The listing builds one solid part. Answer for the finished solid, in the listing's coordinates (mm). Face numbers are marked on the shaded views. Give positions to 0.01 mm unless a question says otherwise; leave off trailing zeros. Order: outer loops, then holes, each group sorted by start corner. A loop starts at its lowest first (then second) coordinate and runs counter-clockwise, first axis right, second up. Notation, with made-up numbers: (59.25, 47.25) -> (98.25, 47.25) arc R12 ccw to (98.25, 56.25) -> close; hole circle Ø11 at (12, -1.75). An arc over 180 degrees is marked (long way). Answer as a JSON object with one key per item and string values. Group by question number.
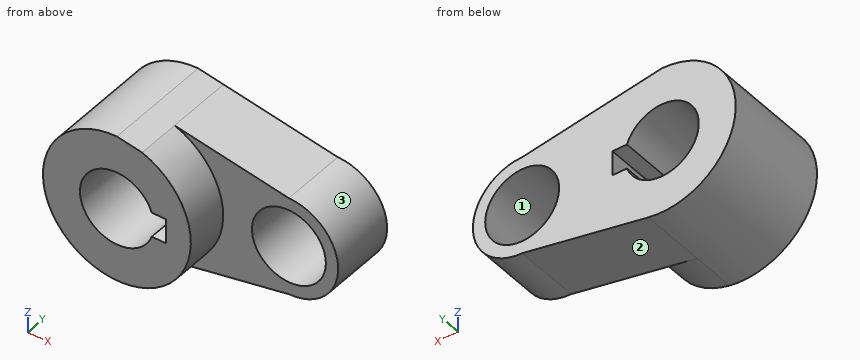
```python
from build123d import *

# Parameters (mm, degrees)
F0_R     = 14.2875
F1_DEPTH = 25.4
F2_DEPTH = 42.21934


with BuildPart() as f1:
    # F0 (on Front) → F1 (new body)
    with BuildSketch(Plane.XZ):
        with BuildLine():
            ThreePointArc((5.2118166453, -28.0956863638), (21.9710978975, -18.2702348693), (28.575, 0))
            ThreePointArc((28.575, 0), (23.4095521288, 16.3866864902), (9.780704698, 26.8489932886))
            Line((9.780704698, 26.8489932886), (0, 28.575))
            ThreePointArc((0, 28.575), (-28.4549192834, -2.6169053435), (5.2118166453, -28.0956863638))
        make_face()
        with BuildLine():
            ThreePointArc((-13.4703841816, 4.7625), (0, 14.2875), (13.4703841816, 4.7625))
            Line((13.4703841816, 4.7625), (19.05, 4.7625))
            Line((19.05, 4.7625), (19.05, -4.7625))
            Line((19.05, -4.7625), (13.4703841816, -4.7625))
            ThreePointArc((13.4703841816, -4.7625), (0, -14.2875), (-13.4703841816, -4.7625))
            Line((-13.4703841816, -4.7625), (-19.05, -4.7625))
            Line((-19.05, -4.7625), (-19.05, 4.7625))
            Line((-19.05, 4.7625), (-13.4703841816, 4.7625))
        make_face(mode=Mode.SUBTRACT)
        with BuildLine():
            ThreePointArc((9.780704698, 26.8489932886), (23.4095521288, 16.3866864902), (28.575, 0))
            ThreePointArc((28.575, 0), (21.9710978975, -18.2702348693), (5.2118166453, -28.0956863638))
            Line((5.2118166453, -28.0956863638), (53.975, -19.05))
            ThreePointArc((53.975, -19.05), (34.925, 0), (53.975, 19.05))
            Line((53.975, 19.05), (9.780704698, 26.8489932886))
        make_face()
        with BuildLine():
            ThreePointArc((73.025, 0), (67.4453841816, 13.4703841816), (53.975, 19.05))
            ThreePointArc((53.975, 19.05), (34.925, 0), (53.975, -19.05))
            ThreePointArc((53.975, -19.05), (67.4453841816, -13.4703841816), (73.025, 0))
        make_face()
        with Locations((53.975, 0)):
            Circle(F0_R, mode=Mode.SUBTRACT)
        with BuildLine():
            ThreePointArc((-13.4703841816, -4.7625), (-14.2875, 0), (-13.4703841816, 4.7625))
            Line((-13.4703841816, 4.7625), (-19.05, 4.7625))
            Line((-19.05, 4.7625), (-19.05, -4.7625))
            Line((-19.05, -4.7625), (-13.4703841816, -4.7625))
        make_face()
    extrude(amount=F1_DEPTH)

    # F0 (on Front) → F2 (join)
    with BuildSketch(Plane.XZ):
        with BuildLine():
            ThreePointArc((5.2118166453, -28.0956863638), (21.9710978975, -18.2702348693), (28.575, 0))
            ThreePointArc((28.575, 0), (23.4095521288, 16.3866864902), (9.780704698, 26.8489932886))
            Line((9.780704698, 26.8489932886), (0, 28.575))
            ThreePointArc((0, 28.575), (-28.4549192834, -2.6169053435), (5.2118166453, -28.0956863638))
        make_face()
        with BuildLine():
            ThreePointArc((-13.4703841816, 4.7625), (0, 14.2875), (13.4703841816, 4.7625))
            Line((13.4703841816, 4.7625), (19.05, 4.7625))
            Line((19.05, 4.7625), (19.05, -4.7625))
            Line((19.05, -4.7625), (13.4703841816, -4.7625))
            ThreePointArc((13.4703841816, -4.7625), (0, -14.2875), (-13.4703841816, -4.7625))
            Line((-13.4703841816, -4.7625), (-19.05, -4.7625))
            Line((-19.05, -4.7625), (-19.05, 4.7625))
            Line((-19.05, 4.7625), (-13.4703841816, 4.7625))
        make_face(mode=Mode.SUBTRACT)
        with BuildLine():
            ThreePointArc((-13.4703841816, -4.7625), (-14.2875, 0), (-13.4703841816, 4.7625))
            Line((-13.4703841816, 4.7625), (-19.05, 4.7625))
            Line((-19.05, 4.7625), (-19.05, -4.7625))
            Line((-19.05, -4.7625), (-13.4703841816, -4.7625))
        make_face()
    extrude(amount=F2_DEPTH)


solid = f1.part
```
(1) Flat-ended cylindrical pins translate along their axes: pin 1 Ø2 at (x, y) = (59.5, -8.5) entering from +Z; pin 2 Ø5 at (y, z) = (-15.5, -16) entering from +X; pin 3 Ø1 at (x, y) = (-18.5, -14.5) entering from -Z. Find the tip coordinate at first contact, or state that the pin passes through.
(2) A cutting plane is placed at A-A (z = 0). State how many separate pieces and enclosed holes the cut face has, and give its area (3 significant figures).
(3) A cutting plane is placed at C-C (x = 15.5). Determine the outline of the cut face in (y, z).
(4) For a pull along Z with two mould halves and no side action, classify the marked faces 1, 2 and 3 as +Z half, -Z half, draft (parallel to the pull), parting line (faces both ways), or undercut.
(5) Find the intervals of material crossed by line 1 along Z through (x, y) = (0, -26) (1 decimal); line 2 along X through (y, z) = (-11.5, 5.5); line 3 along X through (y, z) = (-7, 8), in increasing order. Write a range as [from, to].
Check sheet entries:
{
 "1": {"pin 1": "stops at z = 18.5", "pin 2": "stops at x = 67.42", "pin 3": "stops at z = -22.19"},
 "2": {"separate pieces": "3", "enclosed holes": "0", "area": "1,410 mm2"},
 "3": {"outline": "(-42.22, -24.01) -> (-25.4, -24.01) -> (-25.4, -26.19) -> (0, -26.19) -> (0, -4.76) -> (-42.22, -4.76) -> close; (-42.22, 4.76) -> (0, 4.76) -> (0, 25.84) -> (-25.4, 25.84) -> (-25.4, 24.01) -> (-42.22, 24.01) -> close"},
 "4": {"face 1": "undercut", "face 2": "-Z half", "face 3": "parting line"},
 "5": {"line 1": "z = [-28.6, -14.3], [14.3, 28.6]", "line 2": "x = [-28.04, -13.19], [13.19, 40.79], [67.16, 72.21]", "line 3": "x = [-27.43, -11.84], [11.84, 42.14], [65.81, 71.26]"}
}
